Geometry check sheet. Reference: the model listing, model coordinates, mm. Give positions to 0.01 mm unless a question says otherwise; leave off trailing zeros. One line per item, written item: value. Start each with the question number.
(1) Gauge pin test, flat ends, axial feed: pin 1 Ø5.5 at (x, z) = (90, 30) entering from +Y; pin 2 Ø2.5 at (x, z) = (90, 10) entering from +Y (3 decimals). Record the tip position at first contact, or that the pin passes through.
(2) Draft check along X on faces 1 (the face through (-1, 0.75, 1)), 2 (the face through (-91.65, 0.01, 10.07)). Enter one of: pulls with the +X half, pulls with the -X half, needs draft (parallel to the pull), parting line crosses it, or undercut.
(3) Scan lines: line 1 along Z through (x, y) = (90, 0); line 2 along X through (y, z) = (-0.6, 9). Record each from-to range of solid material in increasing order. Write a range as from..to.
from build123d import *

# Parameters (mm, degrees)
SKETCH_W       = 190
SKETCH_H       = 82
SKETCH_R       = 1.65
PAD_DEPTH      = 0.75
PAD_DEPTH_BACK = 0.75


with BuildPart() as part:
    # Sketch → Pad (new body, two sides)
    with BuildSketch(Plane.XZ) as pad_sk:
        Rectangle(SKETCH_W, SKETCH_H)
        with Locations((90, 30)):
            Circle(SKETCH_R, mode=Mode.SUBTRACT)
        with Locations((90, 10)):
            Circle(SKETCH_R, mode=Mode.SUBTRACT)
        with Locations((90, -30)):
            Circle(SKETCH_R, mode=Mode.SUBTRACT)
        with Locations((90, -10)):
            Circle(SKETCH_R, mode=Mode.SUBTRACT)
        with Locations((-90, 30)):
            Circle(SKETCH_R, mode=Mode.SUBTRACT)
        with Locations((-90, 10)):
            Circle(SKETCH_R, mode=Mode.SUBTRACT)
        with Locations((-90, -30)):
            Circle(SKETCH_R, mode=Mode.SUBTRACT)
        with Locations((-90, -10)):
            Circle(SKETCH_R, mode=Mode.SUBTRACT)
    extrude(amount=PAD_DEPTH)
    extrude(pad_sk.sketch, amount=-PAD_DEPTH_BACK)


solid = part.part
Calculated:
1. pin 1: stops at y = 0.75
1. pin 2: passes through
2. face 1: needs draft
2. face 2: undercut
3. line 1: z = -41..-31.65, -28.35..-11.65, -8.35..8.35, 11.65..28.35, 31.65..41
3. line 2: x = -95..-91.31, -88.69..88.69, 91.31..95
